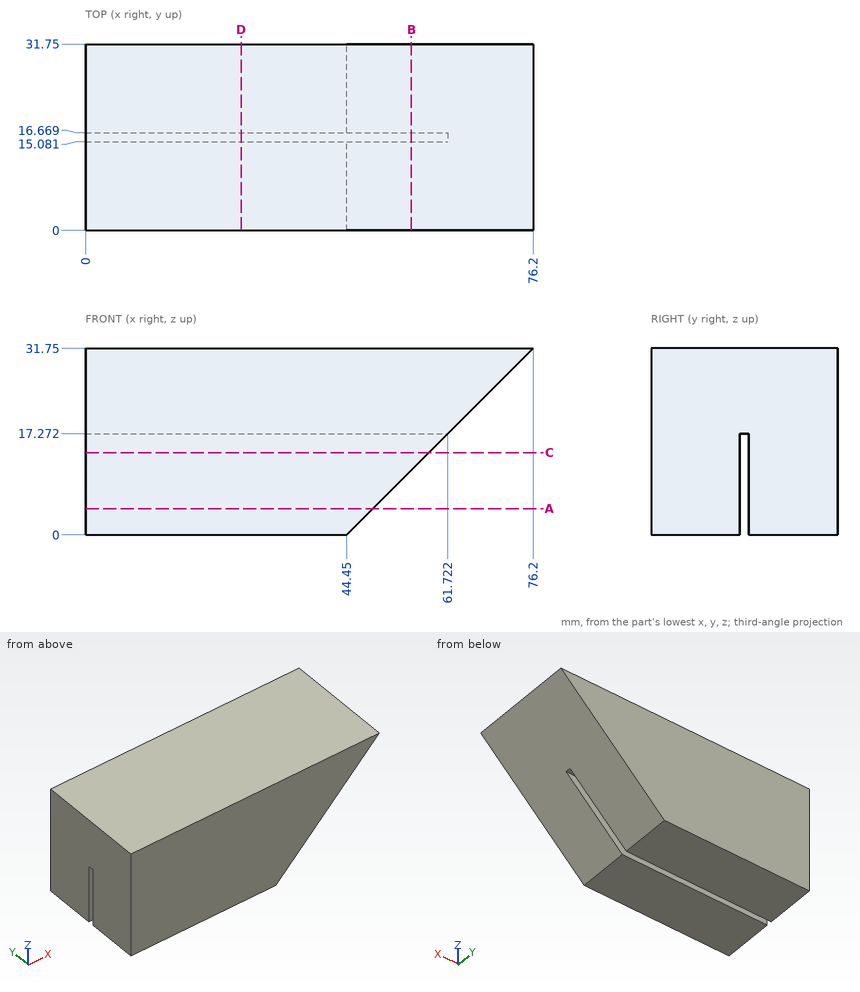
Geometry: see drawing. Coordinates: mm, zero at the bounding-box minimum. Coordinates: 2 decimals unless noted, no trailing zeros. Loops run counter-clockwise (first coordinate to the right, second up) from the corner with the lowest first, then second, coordinate; pieces in that order, holes last.
Q1. Cut plane D-D (x = 26.5). Output: boundary loops of the cut face in (y, z).
Q2. Contact query for flat-ended pins moving along their axis: pin 1 (4 mm diameter, centred on y = 8.5, z = 28, fed in from +X); pin 2 (0.5 mm diameter, centred on x = 39, y = 16, fed in from -Z); pin 3 (1 mm diameter, centred on y = 16.5, z = 11.5, fed in from +X). Output: stop coordinate, or through.
Q3. Cut plane C-C (z = 14). Output: boundary loops of the cut face in (x, y).
Q4. Cut plane B-B (x = 55.5). Output: boundary loops of the cut face in (y, z).
Q5. Cut plane A-A (z = 4.5). Output: boundary loops of the cut face in (x, y).
Q6. Material intervals for line 1 (Y direction, x = 4, z = 6); line 2 (Z direction, x = 9, y = 16); line 3 (X direction, y = 11, z = 4), sorted ascending.
Working result:
1. outline: (0, 0) - (15.08, 0) - (15.08, 17.27) - (16.67, 17.27) - (16.67, 0) - (31.75, 0) - (31.75, 31.75) - (0, 31.75) - close
2. pin 1: stops at x = 74.45
2. pin 2: stops at z = 17.27
2. pin 3: stops at x = 56.42
3. outline: (0, 0) - (58.45, 0) - (58.45, 15.08) - (0, 15.08) - close; (0, 16.67) - (58.45, 16.67) - (58.45, 31.75) - (0, 31.75) - close
4. outline: (0, 11.05) - (15.08, 11.05) - (15.08, 17.27) - (16.67, 17.27) - (16.67, 11.05) - (31.75, 11.05) - (31.75, 31.75) - (0, 31.75) - close
5. outline: (0, 0) - (48.95, 0) - (48.95, 15.08) - (0, 15.08) - close; (0, 16.67) - (48.95, 16.67) - (48.95, 31.75) - (0, 31.75) - close
6. line 1: y = 0 to 15.08, 16.67 to 31.75
6. line 2: z = 17.27 to 31.75
6. line 3: x = 0 to 48.45
